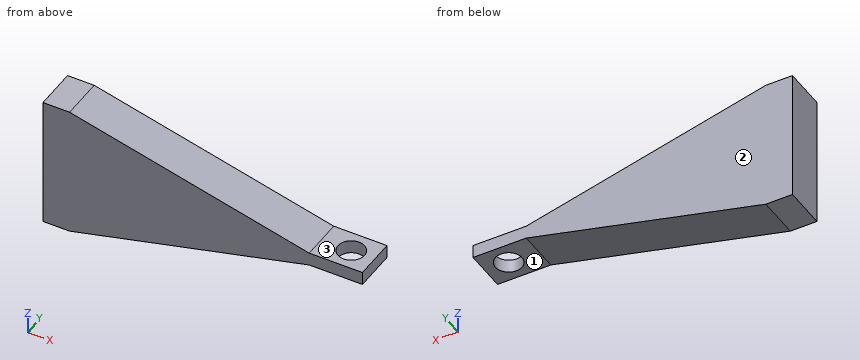
from build123d import *

# Parameters (mm, degrees)
F1_DEPTH = 5.08
F2_W     = 10.16
F2_H     = 3.175
F3_DEPTH = 12.7
F4_R     = 3.175
F5_DEPTH = 25.4


with BuildPart() as f1:
    # F0 (on Front) → F1 (new body, symmetric)
    with BuildSketch(Plane.XZ):
        Polygon((-34.925, -15.875), (-28.575, -15.875), (28.575, -1.5875), (28.575, 1.5875), (-28.575, 15.875), (-34.925, 15.875), align=None)
    extrude(amount=F1_DEPTH, both=True)

    # F2 (on face) → F3 (join)
    with BuildSketch(Plane.YZ.offset(28.575)):
        Rectangle(F2_W, F2_H)
    extrude(amount=F3_DEPTH)

    # F4 (on face) → F5 (cut)
    with BuildSketch(Plane.XY.offset(1.5875)):
        with Locations((35.682857, 0)):
            Circle(F4_R)
    extrude(amount=-F5_DEPTH, mode=Mode.SUBTRACT)


solid = f1.part
Geometry check sheet. Reference: the model listing, model coordinates, mm. Face numbers are marked on the shaded views. A direction names the side the tool comes from. Round coordinates to 2 decimals unless told otherwise and drop trailing zeros. Order: outer loops, then holes, each group sorted by start corner. A loop starts at its lowest first (then second) coordinate and runs counter-clockwise, first axis right, second up. Notation, with made-up numbers: (0, -2) - (41, -2) arc R17 ccw to (41, 29) - close; hole circle Ø3 at (62, -24.5). An arc over 180 degrees is marked (long way). One line per question, with ' | ' between items. Start each with the question number.
(1) Sectioned sample at C-C on x = 11.5. Record the cut outline in (y, z).
(2) Sectioned sample at A-A on y = 0. Record the cut outline in (x, z) (1 decimal).
(3) Sectioned sample at B-B on z = 0.5. Record the cut outline in (x, y) (3 decimals).
(4) Access from +Z, -Z, +X, -X, +Y, -Y to the whole of each face (thin tool, end or side, straight path). Record for the marked faces 1, 2 and 3.
(5) Sectioned sample at D-D on z = 5. Record the cut outline in (x, y) (3 decimals).
(6) Depth check by flat-ended pin: pin 1 Ø4 at (x, y) = (7, 0) entering from -Z; pin 2 Ø2 at (x, y) = (-20, -1) entering from -Z; pin 3 Ø10 at (x, z) = (17, 11) entering from +Y (3 decimals); pin 4 Ø3 at (x, y) = (36.5, -1.5) entering from +Z. Enter the tip coordinate at first touch or a pass-through.
(7) Thickness scan on L1, parallel to Z at x = 31, y = 4.25; L2, parallel to X at y = 0.5, z = -1 (3 decimals); L3, parallel to Z at x = -4, y = -4. Record the ranges inside material, lowest first. Write a range as [from, to].
Conclusion:
1) outline: (-5.08, -5.86) - (5.08, -5.86) - (5.08, 5.86) - (-5.08, 5.86) - close
2) outline: (-34.9, -15.9) - (-28.6, -15.9) - (28.6, -1.6) - (32.5, -1.6) - (32.5, 1.6) - (28.6, 1.6) - (-28.6, 15.9) - (-34.9, 15.9) - close; (38.9, -1.6) - (41.3, -1.6) - (41.3, 1.6) - (38.9, 1.6) - close
3) outline: (-34.925, -5.08) - (41.275, -5.08) - (41.275, 5.08) - (-34.925, 5.08) - close; hole circle Ø6.35 at (35.683, 0)
4) face 1: -Z, +X, +Y, -Y | face 2: +Z, -Z, +X, -X, +Y | face 3: +Z, +X, +Y, -Y
5) outline: (-34.925, -5.08) - (14.925, -5.08) - (14.925, 5.08) - (-34.925, 5.08) - close
6) pin 1: stops at z = -7.48 | pin 2: stops at z = -13.98 | pin 3: passes through | pin 4: stops at z = 1.59
7) L1: z = [-1.59, 1.59] | L2: x = [-34.925, 32.547], [38.818, 41.275] | L3: z = [-9.73, 9.73]
